The model under review builds one solid part; all positions refer to its coordinate system, in mm. Face numbers are marked on the shaded views. Round coordinates to 2 decimals unless told otherwise and drop trailing zeros. Order: outer loops, then holes, each group sorted by start corner. A loop starts at its lowest first (then second) coordinate and runs counter-clockwise, first axis right, second up.
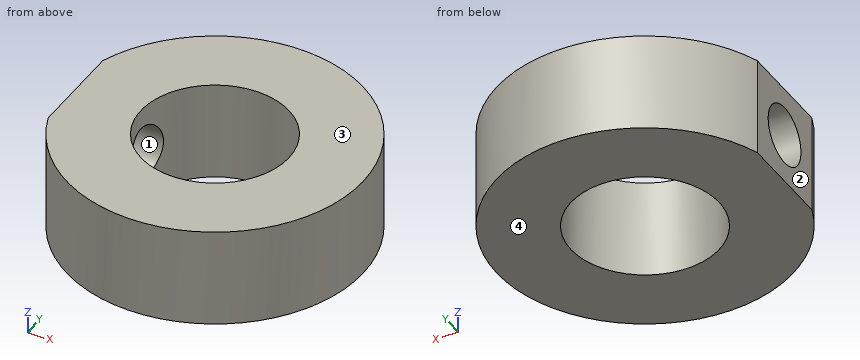
```python
from build123d import *

# Parameters (mm, degrees)
SKIZZE1_R                       = 15
SKIZZE1_R_2                     = 7.5
AUFSATZ_LINEAR_AUSTRAGEN1_DEPTH = 5
SCHNITT_LINEAR_AUSTRAGEN1_DEPTH = 11
SCHNITT_LINEAR_AUSTRAGEN2_REACH = 31.142
SKIZZE3_R                       = 3


with BuildPart() as part:
    # Skizze1 → Aufsatz-Linear austragen1 (new body, symmetric)
    with BuildSketch(Plane.XY):
        Circle(SKIZZE1_R)
        Circle(SKIZZE1_R_2, mode=Mode.SUBTRACT)
    extrude(amount=AUFSATZ_LINEAR_AUSTRAGEN1_DEPTH, both=True)

    # Skizze2 → Schnitt-Linear austragen1 (cut, through all)
    with BuildSketch(Plane.XY.offset(5)):
        with BuildLine():
            Line((-14.142135624, 5), (-14.142135624, -5))
            ThreePointArc((-14.142135624, -5), (-15, 0), (-14.142135624, 5))
        make_face()
    extrude(amount=-SCHNITT_LINEAR_AUSTRAGEN1_DEPTH, mode=Mode.SUBTRACT)

    # Skizze3 → Schnitt-Linear austragen2 (cut, up to next)
    with BuildSketch(Plane.ZY.offset(14.142135624), mode=Mode.PRIVATE) as schnitt_linear_austragen2_sk1:
        Circle(SKIZZE3_R)
    schnitt_linear_austragen2_tool1 = extrude(schnitt_linear_austragen2_sk1.sketch, amount=-SCHNITT_LINEAR_AUSTRAGEN2_REACH, mode=Mode.PRIVATE) & part.part
    add(schnitt_linear_austragen2_tool1.solids().sort_by_distance((-14.142136, 0, 0))[0], mode=Mode.SUBTRACT)


solid = part.part
```
(1) Consider section B-B (y = 0). Write out the cut boundary in (x, z).
Data:
outline: (-14.14, -5) - (-7.5, -5) - (-7.5, -3) - (-14.14, -3) - close; (-14.14, 3) - (-7.5, 3) - (-7.5, 5) - (-14.14, 5) - close; (7.5, -5) - (15, -5) - (15, 5) - (7.5, 5) - close
(2) Insertion check: pin 1 (5.5 mm diameter, centred on y = 0, z = 0, fed in from -X); pin 2 (3 mm diameter, centred on x = -3.5, z = -2, fed in from -Y). Each pin has a flat end and moves straight along its axis. Give the tip position at first contact, or say it passes through.
Data:
pin 1: stops at x = 6.98
pin 2: stops at y = -14.87
(3) Consider section A-A (x = 0). Write out the cut boundary in (y, z), and give its area (3 significant figures).
Data:
outline: (-15, -5) - (-7.5, -5) - (-7.5, 5) - (-15, 5) - close; (7.5, -5) - (15, -5) - (15, 5) - (7.5, 5) - close
area: 150 mm2
(4) To check wall thickness, follow probe 1 along Y at (x, z) = (0, 0.25); probe 2 along Z at (x, y) = (-10, 0); probe 3 along Y at (x, z) = (-10.25, 0). State the ranges of each line that lie inside material, in increasing order.
Data:
probe 1: y = -15 to -7.5, 7.5 to 15
probe 2: z = -5 to -3, 3 to 5
probe 3: y = -10.95 to -3, 3 to 10.95
(5) Consider section C-C (y = -6.25). Write out the cut boundary in (x, z).
Data:
outline: (-13.64, -5) - (-4.15, -5) - (-4.15, 5) - (-13.64, 5) - close; (4.15, -5) - (13.64, -5) - (13.64, 5) - (4.15, 5) - close
(6) Draft analysis for pull direction Z (two halves, no side actions). For the marked faces 1, 2, 3 and 4, state which applies: pulls with the +Z half, pulls with the -Z half, needs draft (parallel to the pull), parting line crosses it, or undercut.
Data:
face 1: undercut
face 2: needs draft
face 3: pulls with the +Z half
face 4: pulls with the -Z half
(7) Consider section D-D (z = 0). Write out the cut boundary in (x, y).
Data:
outline: (-14.14, -5) arc R15 ccw (long way) to (-14.14, 5) - (-14.14, 3) - (-6.87, 3) arc R7.5 cw (long way) to (-6.87, -3) - (-14.14, -3) - close
